Autodesk Inventor part; units mm, degrees
ref_plane "YZ Plane" through (0, 0, 0) normal (1, 0, 0) x (0, 1, 0)
ref_plane "XZ Plane" through (0, 0, 0) normal (0, 1, 0) x (-1, 0, 0)
ref_plane "XY Plane" through (0, 0, 0) normal (0, 0, 1) x (1, 0, 0)
sketch "Profile" plane through (0, 0, 0) normal (0, 1, 0) x (-1, 0, 0)
  line L0 (0, 0) -> (-76.2, 0)
  line L1 (-76.2, 0) -> (-76.2, -50.8)
  line L2 (-76.2, -50.8) -> (0, -50.8)
  line L3 (0, -50.8) -> (0, 0)
  line L4 (0, -25.4) -> (-76.2, -25.4)
  line L5 (-38.1, -50.8) -> (-38.1, 0)
  line L6 (-6.35, -44.45) -> (-69.85, -44.45) construction
  line L7 (-69.85, -44.45) -> (-69.85, -6.35) construction
  line L8 (-69.85, -6.35) -> (-6.35, -6.35) construction
  line L9 (-6.35, -6.35) -> (-6.35, -44.45) construction
  line L10 (-6.35, -44.45) -> (-69.85, -6.35) construction
  line L11 (-69.85, -44.45) -> (-6.35, -6.35) construction
  circle A0 centre (-38.1, -25.4) radius 4.5
  dimension "d0" = 76.2
  dimension "d1" = 50.8
  dimension "d2" = 63.5
  dimension "d3" = 38.1
  dimension "d13" = 9
extrude "Plate1" add sketch "Profile" against normal blind 2
hole "#6 Mounting Hole" at (6.35, 0, -44.45) direction (0, -1, 0) diameter 3.81 end through all countersink diameter 7.0866 countersink angle 82
pattern_sketch "Jack Plate Mounting Holes" of "#6 Mounting Hole" from (6.35, 0, -44.45) copies at (69.85, 0, -44.45) at (69.85, 0, -6.35) at (6.35, 0, -6.35)
hole "Input Jack Hole" at (38.1, 0, -25.4) direction (0, -1, 0) diameter 9.525 end through all
fillet "Corner Round1" radius 3.175 4 edges at (0, -1, -50.8) (76.2, -1, -50.8) (76.2, -1, 0) (0, -1, 0)
equation "\"d11\" = Thickness"
equation "\"d5\" = Thickness"
equation "\"BendRadius\" = Thickness"
equation "\"BendReliefWidth\" = Thickness"
equation "\"BendReliefDepth\" = 0.5 * Thickness"
equation "\"CornerReliefSize\" = 4 * Thickness"
equation "\"MinimumRemnant\" = 2 * Thickness"
equation "\"TransitionRadius\" = BendRadius"
equation "\"JacobiRadiusSize\" = BendRadius"
equation "\"GapSize\" = Thickness"
properties part number "Jack Plate" material "Aluminum 6061"
Input: part model. Units: mm. Frame: model coordinates. Coordinates: 2 decimals unless noted, no trailing zeros. Loops run counter-clockwise (first coordinate to the right, second up) from the corner with the lowest first, then second, coordinate; pieces in that order, holes last. Notation, with made-up numbers: (46, 30) - (52, 30) arc R29 cw to (52, 63) - close; hole circle Ø9 at (54, -1.5). An arc over 180 degrees is marked (long way). Answer in a Markdown table with one row per item.
(1) Cut plane C-C on z = -6.35. Output: boundary loops of the cut face in (x, y) (3 decimals), plus the area to 3 significant figures.
Model answer:
| item | result |
|---|---|
| outline | (0, -2) - (4.445, -2) - (4.445, -1.885) - (2.807, 0) - (0, 0) - close; (8.255, -2) - (67.945, -2) - (67.945, -1.885) - (66.307, 0) - (9.893, 0) - (8.255, -1.885) - close; (71.755, -2) - (76.2, -2) - (76.2, 0) - (73.393, 0) - (71.755, -1.885) - close |
| area | 131 mm² |
(2) Cut plane A-A on z = -25.4. Output: boundary loops of the cut face in (x, y), plus the area to 3 significant figures.
Model answer:
| item | result |
|---|---|
| outline | (0, -2) - (33.34, -2) - (33.34, 0) - (0, 0) - close; (42.86, -2) - (76.2, -2) - (76.2, 0) - (42.86, 0) - close |
| area | 133 mm² |
(3) Material intervals for L1, parallel to X at y = -1.9, z = -44.45 (3 decimals); L2, parallel to Z at x = 69.85, y = -1.95 (3 decimals); L3, parallel to Z at x = 6, y = -0.05, sorted ascending. Write a range as from..to.
Model answer:
| item | result |
|---|---|
| L1 | x = 0..4.445, 8.255..67.945, 71.755..76.2 |
| L2 | z = -50.8..-46.355, -42.545..-8.255, -4.445..0 |
| L3 | z = -50.8..-47.93, -40.97..-9.83, -2.87..0 |
(4) Pin query (flat end, axial travel): P1, Ø5, axis at x = 69.85, z = -44.45, coming from the +Y side. Return the tip coordinate at first contact, or that it passes through.
Model answer:
| item | result |
|---|---|
| P1 | stops at y = -1.2 |
(5) Cut plane D-D on x = 6.35. Output: boundary loops of the cut face in (y, z) (3 decimals), plus the area to 3 significant figures.
Model answer:
| item | result |
|---|---|
| outline | (-2, -50.8) - (0, -50.8) - (0, -47.993) - (-1.885, -46.355) - (-2, -46.355) - close; (-2, -42.545) - (-1.885, -42.545) - (0, -40.907) - (0, -9.893) - (-1.885, -8.255) - (-2, -8.255) - close; (-2, -4.445) - (-1.885, -4.445) - (0, -2.807) - (0, 0) - (-2, 0) - close |
| area | 80.2 mm² |
(6) Mould query, pull axis Z, two halves, no side actions, for faces 1 (the face through (68.069, -1.767, -5.424)), 2 (the face through (0.95, -1.01, -0.91)), 3 (the face through (0.91, -1.01, -49.85)), 4 (the face through (39, -2, -31)). Classes: pulls with the +Z half, pulls with the -Z half, needs draft (parallel to the pull), parting line crosses it, or undercut.
Model answer:
| item | result |
|---|---|
| face 1 | undercut |
| face 2 | pulls with the +Z half |
| face 3 | pulls with the -Z half |
| face 4 | needs draft |
(7) Cut plane B-B on x = 38.1. Output: boundary loops of the cut face in (y, z), plus the area to 4 significant figures.
Model answer:
| item | result |
|---|---|
| outline | (-2, -50.8) - (0, -50.8) - (0, -30.16) - (-2, -30.16) - close; (-2, -20.64) - (0, -20.64) - (0, 0) - (-2, 0) - close |
| area | 82.55 mm² |
